from build123d import *

# Parameters (mm, degrees)
BOSS_EXTRUDE1_DEPTH = 5
SKETCH2_R           = 1.5
CUT_EXTRUDE1_DEPTH  = 4
SKETCH3_R           = 1.27
BOSS_EXTRUDE2_DEPTH = 4
CHAMFER1_SIZE       = 0.254
CHAMFER2_SIZE       = 0.254


with BuildPart() as part:
    # Sketch1 → Boss-Extrude1 (new body)
    with BuildSketch(Plane(origin=(0, 0, 0), x_dir=(1, 0, 0), z_dir=(0, 1, 0))):
        Polygon((2.395673947, -2.502148345), (3.364761004, 0.823640325), (0.969087057, 3.32578867), (-2.395673947, 2.502148345), (-3.364761004, -0.823640325), (-0.969087057, -3.32578867), align=None)
    extrude(amount=BOSS_EXTRUDE1_DEPTH)

    # Sketch2 → Cut-Extrude1 (cut)
    with BuildSketch(Plane(origin=(0, 5, 0), x_dir=(1, 0, 0), z_dir=(0, 1, 0))):
        with Locations(Location((0, 0, 0), (0, 0, 270))):
            Circle(SKETCH2_R)
    extrude(amount=-CUT_EXTRUDE1_DEPTH, mode=Mode.SUBTRACT)

    # Sketch3 → Boss-Extrude2 (add)
    with BuildSketch(Plane.XZ):
        with Locations(Location((0, 0, 0), (0, 0, 90))):
            Circle(SKETCH3_R)
    extrude(amount=BOSS_EXTRUDE2_DEPTH)

    # Chamfer1
    chamfer1_edges = [part.edges().sort_by_distance(p)[0] for p in [
        (0, -4, -1.27),
    ]]
    chamfer(chamfer1_edges, length=CHAMFER1_SIZE)

    # Chamfer2
    chamfer2_edges = [part.edges().sort_by_distance(p)[0] for p in [
        (0, 5, -1.5),
    ]]
    chamfer(chamfer2_edges, length=CHAMFER2_SIZE)


solid = part.part
Could you check a few things on this model? Use its own coordinates, in mm. A direction names the side the tool comes from. Coordinates: 2 decimals unless noted, no trailing zeros. Loops run counter-clockwise (first coordinate to the right, second up) from the corner with the lowest first, then second, coordinate; pieces in that order, holes last.
1. Imagine slicing it at C-C (x = 0). Please give me the cut outline in (y, z), and give its area (3 significant figures).
2. For faces 4 (the face through (-0.05, 0, 1.43)), 5 (the face through (0.45, 2.9, 1.43)), 6 (the face through (0.69, 2.46, 2.92)), which set-ups out of +Z, -Z, +X, -X, +Y, -Y let a thin tool reach every point of the face, with its end or its side?
3. Imagine slicing it at A-A (y = 3). Please give me the cut outline in (x, z).
4. I need wall thicknesses on L1, parallel to Y at x = 1, z = 1; L2, parallel to X at y = 3.05, z = 0; L3, parallel to Y at x = -2.25, z = -0.5. Which ranges of each line are inside material? Lowest first, please.
5. For P1, Ø1.5, axis at x = 2.5, z = -1.5, coming from the -Y side; P2, Ø1, axis at y = 0.5, z = 2, coming from the -X side; P3, Ø1.5, axis at y = 0, z = -1.5, coming from the -X side, each with a flat end and sliding along its axis, tell me the tip position at first contact or that it passes through.
6. Imagine slicing it at D-D (y = -0.5). Please give me the cut outline in (x, z), and give its area (3 significant figures).
7. We'd pull the mould along Z, two halves only. Please class faces 1 (the face through (0, 1, 0)), 2 (the face through (1.4, 5, 1.4)), 3 (the face through (-1.26, -1.85, -0.17)): released by +Z, released by -Z, zero draft, split by the parting line, or undercut.
8. Imagine slicing it at B-B (z = 0). Please give me the cut outline in (x, y), and give its area (3 significant figures).
Computed values:
1. outline: (-4, -1.02) - (-3.75, -1.27) - (0, -1.27) - (0, -3.09) - (5, -3.09) - (5, -1.75) - (4.75, -1.5) - (1, -1.5) - (1, 1.5) - (4.75, 1.5) - (5, 1.75) - (5, 3.09) - (0, 3.09) - (0, 1.27) - (-3.75, 1.27) - (-4, 1.02) - close
1. area: 28.9 mm2
2. face 4: -Y
2. face 5: +Y
2. face 6: +Z, +X, +Y, -Y
3. outline: (-3.36, 0.82) - (-2.4, -2.5) - (0.97, -3.33) - (3.36, -0.82) - (2.4, 2.5) - (-0.97, 3.33) - close; hole circle Ø3 at (0, 0)
4. L1: y = 0 to 1
4. L2: x = -3.12 to -1.5, 1.5 to 3.12
4. L3: y = 0 to 5
5. P1: stops at y = 0
5. P2: stops at x = -2.72
5. P3: stops at x = -2.91
6. outline: circle Ø2.54 at (0, 0)
6. area: 5.07 mm2
7. face 1: undercut
7. face 2: zero draft
7. face 3: split by the parting line
8. outline: (-3.12, 0) - (-1.27, 0) - (-1.27, -3.75) - (-1.02, -4) - (1.02, -4) - (1.27, -3.75) - (1.27, 0) - (3.12, 0) - (3.12, 5) - (1.75, 5) - (1.5, 4.75) - (1.5, 1) - (-1.5, 1) - (-1.5, 4.75) - (-1.75, 5) - (-3.12, 5) - close
8. area: 29.3 mm2
